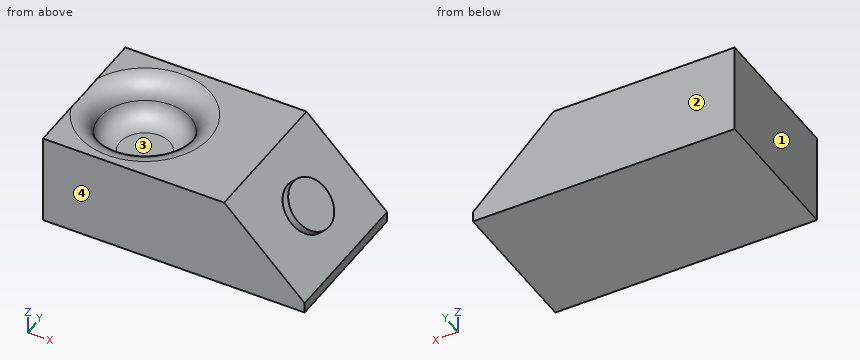
from build123d import *

# Parameters (mm, degrees)
F0_W     = 165.2496345341
F0_H     = 91.986246407
F1_DEPTH = 57.404
F2_R     = 28.4210411612
F3_DEPTH = 25.4
F5_SIZE  = 50.8
F6_R     = 16.0842611484
F7_DEPTH = 5


# Not quite as in the source:
# - a fillet or chamfer that OpenCascade refuses, or shapes differently, is made with other operations: its cross-section is extruded or revolved along the edge and cut away or added


with BuildPart() as f1:
    # F0 (on Top) → F1 (new body)
    with BuildSketch(Plane.XY):
        with Locations((-43.7887068838, 9.0369544923)):
            Rectangle(F0_W, F0_H)
    extrude(amount=F1_DEPTH)

    # F2 (on face) → F3 (cut)
    with BuildSketch(Plane.XY.offset(57.404)):
        with Locations((-87.9544317722, 8.8456757367)):
            Circle(F2_R)
    extrude(amount=-F3_DEPTH, mode=Mode.SUBTRACT)

    # F4: fillet of radius 12.7 on 2 edges, made by hand

    # F4_s1 → F4_t2 (revolve)
    with BuildSketch(Plane.XZ.offset(-8.8456757367)):
        with BuildLine():
            ThreePointArc((-59.5333906111, 44.704), (-63.25313449, 35.7237438789), (-72.2333906111, 32.004))
            Line((-72.2333906111, 32.004), (-59.5333906111, 32.004))
            Line((-59.5333906111, 32.004), (-59.5333906111, 44.704))
        make_face()
    revolve(axis=Axis((-87.9544317722, 8.8456757367, 32.004), (0, 0, 1)))

    # F4_s3 → F4_t4 (revolve, cut)
    with BuildSketch(Plane.XZ.offset(-8.8456757367)):
        with BuildLine():
            ThreePointArc((-46.8333906111, 57.404), (-55.8136467322, 53.6842561211), (-59.5333906111, 44.704))
            Line((-59.5333906111, 44.704), (-59.5333906111, 57.404))
            Line((-59.5333906111, 57.404), (-46.8333906111, 57.404))
        make_face()
    revolve(axis=Axis((-87.9544317722, 8.8456757367, 57.404), (0, 0, 1)), mode=Mode.SUBTRACT)

    # F5
    f5_edges = [f1.edges().sort_by_distance(p)[0] for p in [
        (38.83611, 9.036954, 57.404),
    ]]
    chamfer(f5_edges, length=F5_SIZE)

    # F6 (on face) → F7 (join)
    with BuildSketch(Plane(origin=(22.7200551916, 0, 22.7200551916), x_dir=(0, 1, 0), z_dir=(0.7071067812, 0, 0.7071067812))):
        with Locations((9.0369544923, 13.1294806603)):
            Circle(F6_R)
    extrude(amount=F7_DEPTH)


solid = f1.part
Verification items for the finished model (mm, model axes). Face numbers are marked on the shaded views. Give positions to 0.01 mm unless a question says otherwise; leave off trailing zeros. Loops run counter-clockwise (first coordinate to the right, second up) from the corner with the lowest first, then second, coordinate; pieces in that order, holes last.
1) Draft check along Y on the marked faces 1, 2, 3 and 4. Enter one of: pulls with the +Y half, pulls with the -Y half, needs draft (parallel to the pull), parting line crosses it, or undercut.
2) Thickness scan on line 1 along X through (y, z) = (-24.5, 52.5); line 2 along Y through (x, z) = (-74, 55); line 3 along X through (y, z) = (25, 38). Record the ranges inside material, lowest first.
3) Sectioned sample at A-A, the plane z = 48.5. Enter the section's corners in (x, y), then the cut area to 3 significant figures.
4) Depth check by flat-ended pin: pin 1 Ø10 at (x, y) = (-85.5, 36) entering from +Z; pin 2 Ø1 at (y, z) = (23, 29.5) entering from +X; pin 3 Ø12 at (y, z) = (15.5, 32) entering from +X. Enter the tip coordinate at first touch or a pass-through.
5) Sectioned sample at B-B, the plane z = 18. Enter the section's corners in (x, y), then the cut area to 3 significant figures.
Answers:
1. face 1: needs draft
1. face 2: pulls with the +Y half
1. face 3: undercut
1. face 4: pulls with the -Y half
2. line 1: x = -126.41 to -7.06
2. line 2: y = -36.96 to -21.81, 39.51 to 55.03
2. line 3: x = -126.41 to -108.97, -66.94 to 7.44
3. outline: (-126.41, -36.96) - (-3.06, -36.96) - (-3.06, 55.03) - (-126.41, 55.03) - close; hole circle Ø58 at (-87.95, 8.85)
3. area: 8,700 mm2
4. pin 1: stops at z = 53.81
4. pin 2: stops at x = 23.17
4. pin 3: stops at x = 26.51
5. outline: (-126.41, -36.96) - (27.44, -36.96) - (27.44, 55.03) - (-126.41, 55.03) - close
5. area: 14,200 mm2
